Geometry: final body of the model. Coordinates: model frame, mm. A direction names the side the tool comes from. Round coordinates to 2 decimals unless told otherwise and drop trailing zeros. Order: outer loops, then holes, each group sorted by start corner. A loop starts at its lowest first (then second) coordinate and runs counter-clockwise, first axis right, second up. Notation, with made-up numbers: M -21.5,-3.75 L 26.5,-3.75 A10 ccw 26.5,14.25 Z; hole C 46.5,55.5 d1. An arc over 180 degrees is marked long. Return JSON: item names as keys, results as strings. Group by question number.
Q1. Ray query, probe 1 along Y at (x, z) = (0, 1.55); probe 2 along Y at (x, z) = (0, 3.25); probe 3 along X at (y, z) = (-0.75, 1.55). Return the intervals inside material, ascending.
Q2. Cut plane B-B on y = 0. Output: boundary loops of the cut face in (x, z), and give its area (3 significant figures).
Q3. Cut plane A-A on z = 1.2. Output: boundary loops of the cut face in (x, y), and give its area (3 significant figures).
Q4. Access query for faces 5 (the face through (-0.585, -2.636, 3.824)), 6 (the face through (10.199, 3.714, 1.134)). Directions: +Z, -Z, +X, -X, +Y, -Y. A direction counts if a zero-diameter tool reaches every point of the face in a straight line with its end or side. Return the directions, or none.
Q5. Cut plane C-C on y = -4. Output: boundary loops of the cut face in (x, z).
Q6. Mould query, pull axis X, two halves, no side actions, for faces 1 (the face through (-1.4, 0.06, 1.06)), 2 (the face through (0, -3, 0)), 3 (the face through (19, 0, 1)), 4 (the face through (1.2, -1.2, 2.1)). Classes: released by +X, released by -X, zero draft, split by the parting line, or undercut.
Q7. Contact query for flat-ended pins moving along their axis: pin 1 (3 mm diameter, centred on x = 8, y = 0.5, fed in from -Z); pin 2 (1.6 mm diameter, centred on x = 0.5, y = 1, fed in from +Z); pin 3 (3 mm diameter, centred on y = -2.5, z = 2.5, fed in from -X); pin 4 (1.5 mm diameter, centred on x = 4.5, z = 3, fed in from +Y). Output: stop coordinate, or through.
Q8. Cut plane D-D on x = -15.5. Output: boundary loops of the cut face in (y, z).
Autodesk Inventor part; units mm, degrees
ref_plane "YZ Plane" through (0, 0, 0) normal (1, 0, 0) x (0, 1, 0)
ref_plane "XY Plane" through (0, 0, 0) normal (0, 0, 1) x (1, 0, 0)
sketch "Sketch1" plane through (0, 0, 0) normal (0, 0, 1) x (1, 0, 0)
  arc A0 (-16.6686, 2.7179) -> (-16.6686, -2.7179) centre (-16.25, 0) ccw
  arc A1 (16.6686, -2.7179) -> (16.6686, 2.7179) centre (16.25, 0) ccw
  line L0 (-3.9085, 4.6833) -> (-16.6686, 2.7179)
  line L1 (-3.9085, -4.6833) -> (-16.6686, -2.7179)
  line L2 (3.9085, -4.6833) -> (16.6686, -2.7179)
  line L3 (3.9085, 4.6833) -> (16.6686, 2.7179)
  arc A2 (-3.9085, -4.6833) -> (3.9085, -4.6833) centre (0, 0) ccw
  arc A3 (3.9085, 4.6833) -> (-3.9085, 4.6833) centre (0, 0) ccw
  point P0 (0, 4.6833)
  dimension "d2" = 5.5
  dimension "d3" = 5.5
extrude "Extrusion1" add sketch "Sketch1" along normal blind 2.3
sketch "Sketch2" plane through (0, 0, 2.3) normal (0, 0, 1) x (1, 0, 0)
  arc A0 (-3.9085, -4.6833) -> (3.9085, -4.6833) centre (0, 0) ccw
  circle A1 centre (0, 0) radius 4.45
  dimension "d6" = 8.9
extrude "Extrusion2" add sketch "Sketch2" along normal blind 3.2
sketch "Sketch3" plane through (0, 0, 5.5) normal (0, 0, 1) x (1, 0, 0)
  circle A0 centre (0, 0) radius 4.45
  circle A1 centre (0, 0) radius 2.7
  dimension "d9" = 5.4
extrude "Extrusion3" cut sketch "Sketch3" against normal blind 3.4 contours A1
sketch "Sketch4" plane through (0, 0, 2.1) normal (0, 0, 1) x (1, 0, 0)
  circle A0 centre (0, 0) radius 2.7
  circle A1 centre (0, 0) radius 1.4
  dimension "d12" = 2.8
extrude "Extrusion4" cut sketch "Sketch4" against normal blind 3.4 contours A1
ref_plane "ConstraintPlane" through (0, 0, 0) normal (0, 1, 0) x (-1, 0, 0)
properties part number "MG996RHorn"
Result sheet:
{
 "1": {"probe 1": "y = -6.1 to -1.4, 1.4 to 6.1", "probe 2": "y = -4.45 to -2.7, 2.7 to 4.45", "probe 3": "x = -18.9 to -1.18, 1.18 to 18.9"},
 "2": {"outline": "M -19,0 L -1.4,0 L -1.4,2.1 L -2.7,2.1 L -2.7,5.5 L -4.45,5.5 L -4.45,2.3 L -19,2.3 Z; M 1.4,0 L 19,0 L 19,2.3 L 4.45,2.3 L 4.45,5.5 L 2.7,5.5 L 2.7,2.1 L 1.4,2.1 Z", "area": "91.6 mm²"},
 "3": {"outline": "M -16.67,-2.72 L -3.91,-4.68 A6.1 ccw 3.91,-4.68 L 16.67,-2.72 A2.75 ccw 16.67,2.72 L 3.91,4.68 A6.1 ccw -3.91,4.68 L -16.67,2.72 A2.75 ccw Z; hole C 0,0 d2.8", "area": "290 mm²"},
 "4": {"face 5": "+Z", "face 6": "+Z, -Z, +X, +Y"},
 "5": {"outline": "M -8.34,0 L 8.34,0 L 8.34,2.3 L 1.95,2.3 L 1.95,5.5 L -1.95,5.5 L -1.95,2.3 L -8.34,2.3 Z"},
 "6": {"face 1": "undercut", "face 2": "zero draft", "face 3": "released by +X", "face 4": "undercut"},
 "7": {"pin 1": "stops at z = 0", "pin 2": "stops at z = 2.1", "pin 3": "stops at x = -18.81", "pin 4": "stops at y = 4.63"},
 "8": {"outline": "M -2.9,0 L 2.9,0 L 2.9,2.3 L -2.9,2.3 Z"}
}
